from build123d import *

# Parameters (mm, degrees)
SKETCH2_W           = 14.35
SKETCH2_H           = 14.35
BOSS_EXTRUDE1_DEPTH = 3
BOSS_EXTRUDE2_DEPTH = 5
SKETCH4_W           = 14.35
SKETCH4_H           = 14.35
SKETCH4_W_2         = 10
SKETCH4_H_2         = 7.368246804
CUT_EXTRUDE1_DEPTH  = 1
FILLET1_R           = 0.5


with BuildPart() as part:
    # Sketch2 → Boss-Extrude1 (new body)
    with BuildSketch(Plane(origin=(0, 0, 0), x_dir=(1, 0, 0), z_dir=(0, 1, 0))):
        Rectangle(SKETCH2_W, SKETCH2_H)
    extrude(amount=BOSS_EXTRUDE1_DEPTH)

    # Sketch3 → Boss-Extrude2 (add, symmetric)
    with BuildSketch(Plane(origin=(0, 0, 0), x_dir=(0, 0, -1), z_dir=(1, 0, 0))):
        Polygon((-1.75, 0), (1.75, 0), (3.684123402, -3.35), (-3.684123402, -3.35), align=None)
    extrude(amount=BOSS_EXTRUDE2_DEPTH, both=True)

    # Sketch4 → Cut-Extrude1 (cut)
    with BuildSketch(Plane.XZ):
        Rectangle(SKETCH4_W, SKETCH4_H)
        Rectangle(SKETCH4_W_2, SKETCH4_H_2, mode=Mode.SUBTRACT)
    extrude(amount=-CUT_EXTRUDE1_DEPTH, mode=Mode.SUBTRACT)

    # Fillet1
    fillet1_edges = [part.edges().sort_by_distance(p)[0] for p in [
        (0, -3.35, -3.684123402),
        (0, 0, -1.75),
        (0, 0, 1.75),
        (0, -3.35, 3.684123402),
    ]]
    fillet(fillet1_edges, radius=FILLET1_R)


solid = part.part
CAD build for the part. Positions are in the model's coordinates, mm. A direction names the side the tool comes from. Give positions to 0.01 mm unless a question says otherwise; leave off trailing zeros. Order: outer loops, then holes, each group sorted by start corner. A loop starts at its lowest first (then second) coordinate and runs counter-clockwise, first axis right, second up. Notation, with made-up numbers: (70.5, 13) -> (120.5, 13) arc R30 cw to (120.5, 48) -> close; hole circle Ø4 at (5, -0.75). An arc over 180 degrees is marked (long way). Return JSON: item names as keys, results as strings.
Q1. Saw through at C-C (y = 0.25). Write the cut outline in (x, z), then the cut area to 3 significant figures.
Working result:
{"outline": "(-5, -3.68) -> (5, -3.68) -> (5, 3.68) -> (-5, 3.68) -> close", "area": "73.7 mm²"}
Q2. Drill centre lines: line 1 (Y direction, x = -0.75, z = 5); line 2 (Y direction, x = 0.25, z = 2.25); line 3 (X direction, y = -0.5, z = -1). Where is each one in solid material? Low to high.
Working result:
{"line 1": "1 to 3", "line 2": "-3.35 to -0.87, -0.16 to 3", "line 3": "-5 to 5"}
Q3. Saw through at D-D (z = 3.5). Write the cut outline in (x, y) (3 decimals), then the cut area to 3 significant figures.
Working result:
{"outline": "(-7.175, 1) -> (-5, 1) -> (-5, 0) -> (5, 0) -> (5, 1) -> (7.175, 1) -> (7.175, 3) -> (-7.175, 3) -> close", "area": "38.7 mm²"}
Q4. Which spindle directions (+Z, -Z, +X, -X, +Y, -Y) get a long thin tool onto all of the face, cutting with end or side? Do faces 4 (the face through (0, 0, -3)), 5 (the face through (-0.1, 0.5, 3.684)), 6 (the face through (-5, -1, 0)), 7 (the face through (0, 0, 3)). Say none if no direction does.
Working result:
{"face 4": "-Z, +X, -X", "face 5": "+Z, +X, -X, -Y", "face 6": "+Z, -Z, -X, -Y", "face 7": "+Z, +X, -X"}
Q5. Mould opens along Y. For faces 1 (the face through (-0.1, 0.5, -3.684)), 2 (the face through (0, 3, 0)), 3 (the face through (0.07, -1.688, 2.725)) say: pulls with the +Y half, pulls with the -Y half, needs draft (parallel to the pull), parting line crosses it, or undercut.
Working result:
{"face 1": "needs draft", "face 2": "pulls with the +Y half", "face 3": "undercut"}
Q6. Saw through at A-A (z = 1.25). Write the cut outline in (x, y) (3 decimals).
Working result:
{"outline": "(-7.175, 1) -> (-5, 1) -> (-5, -3.35) -> (5, -3.35) -> (5, 1) -> (7.175, 1) -> (7.175, 3) -> (-7.175, 3) -> close"}
Q7. Flat gauge pins, fed straight in: pin 1 (3 mm diameter, centred on x = -2, y = -2, fed in from -Z); pin 2 (1.3 mm diameter, centred on y = -0.5, z = -0.5, fed in from -X); pin 3 (2 mm diameter, centred on y = -1.5, z = 1, fed in from +X). Where does each tip first touch, or does it go through?
Working result:
{"pin 1": "z = -3.32", "pin 2": "x = -5", "pin 3": "x = 5"}
Q8. Saw through at B-B (x = 0). Write the cut outline in (y, z) (3 decimals), then the cut area to 3 significant figures.
Working result:
{"outline": "(-3.35, -2.818) arc R0.5 ccw to (-2.6, -3.251) -> (-0.75, -2.183) arc R0.5 cw to (0, -2.616) -> (0, -3.684) -> (1, -3.684) -> (1, -7.175) -> (3, -7.175) -> (3, 7.175) -> (1, 7.175) -> (1, 3.684) -> (0, 3.684) -> (0, 2.616) arc R0.5 cw to (-0.75, 2.183) -> (-2.6, 3.251) arc R0.5 ccw to (-3.35, 2.818) -> close", "area": "54.3 mm²"}
